Here's how the part is built. I have some questions about the finished solid (model axes, mm). Coordinates: 2 decimals unless noted, no trailing zeros. Write each loop counter-clockwise with the first axis right and the second up, starting at its lowest first coordinate (ties: lowest second). Pieces come first, ordered by that corner, then holes.
Item 1: Please list where these lines run through material, in increasing order: line 1 (Z direction, x = 10.2, y = 0); line 2 (Y direction, x = -11.8, z = 101.6); line 3 (X direction, y = -4, z = -9) (3 decimals).
Item 2: I want a section at C-C (z = -4.5). Please give me the cut outline in (x, y) (3 decimals), and give its area (3 significant figures).
Item 3: I want a section at A-A (x = -7.5). Please give me the cut outline in (y, z) (3 decimals).
Item 4: I want a section at D-D (z = 76.2). Please give me the cut outline in (x, y) (3 decimals).
Item 5: I want a section at B-B (y = -19.5). Please give me the cut outline in (x, z) (3 decimals).
Item 6: I'm going to push flat-ended pins straight in: P1, Ø4.5, axis at y = 0, z = -57.15, coming from the -X side; P2, Ø6.5, axis at x = 0, z = 50.8, coming from the +Y side. Where does each tip first touch, or does it pass through?
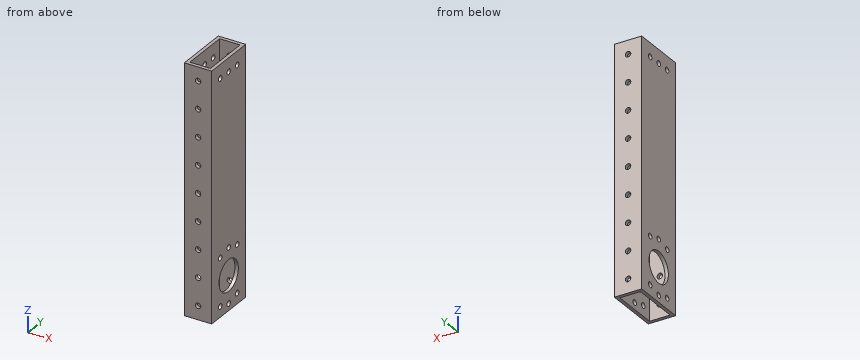
Autodesk Inventor part; units mm, degrees
ref_plane "YZ Plane" through (0, 0, 0) normal (1, 0, 0) x (0, 1, 0)
ref_plane "XZ Plane" through (0, 0, 0) normal (0, 1, 0) x (-1, 0, 0)
ref_plane "XY Plane" through (0, 0, 0) normal (0, 0, 1) x (1, 0, 0)
sketch "Sketch1" plane through (0, 0, 0) normal (0, 0, 1) x (1, 0, 0)
  line L0 (-12.7, -25.4) -> (12.7, -25.4)
  line L1 (12.7, -25.4) -> (12.7, 25.4)
  line L2 (12.7, 25.4) -> (-12.7, 25.4)
  line L3 (-12.7, 25.4) -> (-12.7, -25.4)
  line L4 (-12.7, -25.4) -> (12.7, 25.4) construction
  line L5 (12.7, -25.4) -> (-12.7, 25.4) construction
  line L6 (-9.525, 22.225) -> (9.525, 22.225)
  line L7 (9.525, 22.225) -> (9.525, -22.225)
  line L8 (9.525, -22.225) -> (-9.525, -22.225)
  line L9 (-9.525, -22.225) -> (-9.525, 22.225)
  point P0 (0, 0)
  dimension "width" = 25.4
  dimension "height" = 50.8
  dimension "thickness" = 3.175
extrude "Extrusion1" add sketch "Sketch1" along normal mid plane 228.6
sketch "Sketch3" plane through (-12.7, -25.4, -114.3) normal (-1, 0, 0) x (0, 0, 1)
  circle A0 centre (25.4, 25.4) radius 14.2875
  line L0 (0, 0) -> (0, 50.8)
  point P0 (114.3, 25.4)
  dimension "d8" = 28.575
  dimension "d9" = 25.4
extrude "Extrusion3" [suppressed]
sketch "Sketch4" plane through (-12.7, 25.4, 114.3) normal (0, 1, 0) x (1, 0, 0)
  line L0 (0, 228.6) -> (0, 0)
  line L1 (25.4, 0) -> (0, 0)
  line L2 (25.4, 228.6) -> (25.4, 0)
  line L3 (0, 228.6) -> (25.4, 228.6) construction
  line L4 (0, 228.6) -> (0, 0) construction
  line L5 (25.4, 228.6) -> (25.4, 0) construction
  line L6 (0, 0) -> (25.4, 0) construction
  line L7 (25.4, 0) -> (0, 25.4)
  line L8 (0, 25.4) -> (0, 0)
  line L9 (0, 0) -> (25.4, 0)
  point P0 (12.7, 114.3)
  point P1 (0, 25.4)
  dimension "d17" = 45
extrude "Extrusion4" [suppressed]
sketch "Sketch5" plane through (-12.7, 25.4, -114.3) normal (0, 1, 0) x (1, 0, 0)
  line L0 (0, 0) -> (25.4, 0) construction
  line L1 (25.4, 0) -> (25.4, -228.6) construction
  line L2 (0, -228.6) -> (0, 0) construction
  line L3 (25.4, -228.6) -> (0, -228.6)
  point P0 (12.7, -114.3)
  point P1 (12.7, -12.7)
  point P2 (12.7, 0)
  dimension "d18" = 12.7
hole "Hole1" at (0, 25.4, -101.6) direction (0, -1, 0) diameter 5.1054 end through all
pattern_linear "Rectangular Pattern1" count 9 spacing 25.4 along (0, 0, 1) of "Hole1"
sketch "Sketch6" plane through (-12.7, 25.4, 114.3) normal (0, 1, 0) x (1, 0, 0)
  circle A0 centre (12.7, 38.1) radius 2.5527 construction
  circle A1 centre (12.7, 63.5) radius 2.5527 construction
  circle A2 centre (12.7, 88.9) radius 2.5527 construction
  circle A3 centre (12.7, 114.3) radius 2.5527 construction
  circle A4 centre (12.7, 139.7) radius 2.5527 construction
  circle A5 centre (12.7, 165.1) radius 2.5527 construction
  circle A6 centre (12.7, 190.5) radius 2.5527 construction
  circle A7 centre (12.7, 215.9) radius 2.5527 construction
  line L0 (0, 228.6) -> (25.4, 228.6) construction
  line L1 (25.4, 228.6) -> (25.4, 0) construction
  line L2 (25.4, 0) -> (0, 0) construction
  line L3 (0, 0) -> (0, 228.6) construction
  line L4 (25.4, 0) -> (25.4, 25.4)
  line L5 (25.4, 25.4) -> (0, 0)
  line L6 (0, 0) -> (25.4, 0)
  circle A8 centre (12.7, 12.7) radius 2.5527
  dimension "d29" = 45
extrude "Extrusion5" [suppressed]
sketch "Sketch7" plane through (12.7, -25.4, 114.3) normal (1, 0, 0) x (0, 0, -1)
  line L0 (228.6, 50.8) -> (228.6, 0) construction
  line L1 (228.6, 0) -> (0, 0) construction
  line L2 (0, 0) -> (0, 50.8) construction
  line L3 (0, 50.8) -> (228.6, 50.8) construction
  point P0 (114.3, 25.4)
  point P1 (12.7, 38.1)
  point P2 (12.7, 25.4)
  point P3 (12.7, 12.7)
  point P4 (0, 25.4)
  dimension "d32" = 12.7
  dimension "d33" = 12.7
  dimension "d34" = 12.7
hole "Hole2" at (12.7, 12.7, 101.6) at (12.7, 0, 101.6) at (12.7, -12.7, 101.6) direction (-1, 0, 0) diameter 5.1054 end through all
sketch "Sketch8" plane through (12.7, -25.4, 114.3) normal (1, 0, 0) x (0, 0, -1)
  circle A0 centre (12.7, 25.4) radius 2.5527 construction
  circle A1 centre (12.7, 38.1) radius 2.5527 construction
  circle A2 centre (12.7, 12.7) radius 2.5527 construction
  line L0 (228.6, 50.8) -> (228.6, 0) construction
  line L1 (228.6, 0) -> (0, 0) construction
  line L2 (0, 0) -> (0, 50.8) construction
  line L3 (0, 50.8) -> (228.6, 50.8) construction
  circle A3 centre (196.85, 25.4) radius 23.8125 construction
  circle A4 centre (196.85, 25.4) radius 25.4 construction
  circle A5 centre (196.85, 25.4) radius 50.8 construction
  circle A6 centre (196.85, 25.4) radius 76.2 construction
  point P0 (114.3, 25.4)
  point P1 (220.6625, 25.4)
  point P2 (218.847, 38.1)
  point P3 (208.7562, 46.0222)
  point P4 (184.9437, 46.0222)
  point P5 (173.0375, 25.4)
  point P6 (184.9437, 4.7778)
  point P7 (208.7562, 4.7778)
  point P8 (209.55, 47.397)
  point P9 (196.85, 50.8)
  point P10 (184.15, 47.397)
  point P11 (174.853, 38.1)
  point P12 (171.45, 25.4)
  point P13 (174.853, 12.7)
  point P14 (184.15, 3.403)
  point P15 (196.85, 0)
  point P16 (209.55, 3.403)
  point P17 (218.847, 12.7)
  point P18 (222.25, 25.4)
  dimension "d42" = 47.625
  dimension "d43" = 50.8
  dimension "d44" = 101.6
  dimension "d45" = 152.4
  dimension "d46" = 31.75
  dimension "d49" = 360
  dimension "d53" = 360
hole "Hole3" [suppressed]
hole "Hole4" at (12.7, 12.7, -104.547) at (12.7, 12.7, -60.553) at (12.7, 0, -57.15) at (12.7, -12.7, -60.553) at (12.7, -12.7, -104.547) at (12.7, 0, -107.95) direction (-1, 0, 0) diameter 5.1054 end through all
hole "Hole5" at (12.7, 0, -82.55) direction (-1, 0, 0) diameter 28.956 end through all
properties part number "CL3-001" material "Aluminum 6061"
Answer:
1. line 1: z = -114.3 to -110.5, -105.4 to -97.03, -68.07 to -59.7, -54.6 to 99.05, 104.15 to 114.3
1. line 2: y = -25.4 to -15.25, -10.15 to -2.55, 2.55 to 10.15, 15.25 to 25.4
1. line 3: x = -12.7 to -9.525, 9.525 to 12.7
2. outline: (-12.7, -25.4) - (12.7, -25.4) - (12.7, 25.4) - (-12.7, 25.4) - close; hole (-9.525, -22.225) - (9.525, -22.225) - (9.525, 22.225) - (-9.525, 22.225) - close
2. area: 444 mm2
3. outline: (-25.4, -114.3) - (-22.225, -114.3) - (-22.225, 114.3) - (-25.4, 114.3) - close; (22.225, -114.3) - (25.4, -114.3) - (25.4, 114.3) - (22.225, 114.3) - close
4. outline: (-12.7, -25.4) - (-2.553, -25.4) - (-2.553, -22.225) - (-9.525, -22.225) - (-9.525, 22.225) - (-2.553, 22.225) - (-2.553, 25.4) - (-12.7, 25.4) - close; (2.553, -25.4) - (12.7, -25.4) - (12.7, 25.4) - (2.553, 25.4) - (2.553, 22.225) - (9.525, 22.225) - (9.525, -22.225) - (2.553, -22.225) - close
5. outline: (-12.7, -114.3) - (-9.525, -114.3) - (-9.525, 114.3) - (-12.7, 114.3) - close; (9.525, -114.3) - (12.7, -114.3) - (12.7, 114.3) - (9.525, 114.3) - close
6. P1: passes through
6. P2: stops at y = 25.4
